Check sheet for the modelled part. Datum: model origin and axes. Units: mm. A direction names the side the tool comes from. Round coordinates to 2 decimals unless told otherwise and drop trailing zeros. Write each loop counter-clockwise with the first axis right and the second up, starting at its lowest first coordinate (ties: lowest second). Pieces come first, ordered by that corner, then holes. Notation, with made-up numbers: (-18.5, -17) -> (30.5, -17) arc R13 ccw to (30.5, 0) -> close; hole circle Ø5 at (88, 31). An arc over 180 degrees is marked (long way). Write item = value, one per line.
from build123d import *

# Parameters (mm, degrees)
F_4_0_4_DURCHMESSER_BOHRUNG1_D     = 4
F_4_0_4_DURCHMESSER_BOHRUNG1_DEPTH = 5.001
KREISMUSTER1_COUNT                 = 4


with BuildPart() as part:
    # Skizze1 → Rotation1 (revolve)
    with BuildSketch(Plane.XY):
        Polygon((0, 12.75), (3, 12.75), (3, 9.75), (23, 7.5), (38, 0), (40, 0), (40, 8), (5, 15.5), (5, 25), (0, 25), align=None)
    revolve(axis=Axis((-34.842488806, 0, 0), (1, 0, 0)))

    # Ø4.0 (4) Durchmesser Bohrung1
    with Locations(Plane.ZY):
        with Locations((-19.44, 0)):
            f_4_0_4_durchmesser_bohrung1 = Hole(F_4_0_4_DURCHMESSER_BOHRUNG1_D / 2, depth=F_4_0_4_DURCHMESSER_BOHRUNG1_DEPTH)

    # Kreismuster1: Ø4.0 (4) Durchmesser Bohrung1 ×4 about axis
    kreismuster1_axis = Axis((0, 0, 0), (1, 0, 0))
    for i in range(1, KREISMUSTER1_COUNT):
        add(f_4_0_4_durchmesser_bohrung1.rotate(kreismuster1_axis, i * 360 / KREISMUSTER1_COUNT), mode=Mode.SUBTRACT)


solid = part.part
(1) Access from +Z, -Z, +X, -X, +Y, -Y to the whole of each face (thin tool, end or side, straight path). Record for faces 1 (the flat face through (40, 0, 0)), 2 (the flat face through (3, 6.6, -7.5)).
Worked answers:
face_1 = +Z, -Z, +X, +Y, -Y
face_2 = -X
(2) Sectioned sample at A-A on y = -19.44. Enter the section's corners in (x, z).
Worked answers:
outline = (0, -15.72) -> (5, -15.72) -> (5, -2) -> (0, -2) -> close; (0, 2) -> (5, 2) -> (5, 15.72) -> (0, 15.72) -> close
(3) Sectioned sample at C-C on x = 18.5. Enter the section's corners in (y, z).
Worked answers:
outline = circle Ø25.21 at (0, 0); hole circle Ø16.01 at (0, 0)
(4) Release check for a two-part mould opening along Y. For faces 3 (the flat face through (5, 11.5, -10.8)), 4 (the conical face through (26.144, 10.463, 3.295)), 5 (the cylindrical face through (2.535, 21.287, -0.766)) record: pulls with the +Y half, pulls with the -Y half, needs draft (parallel to the pull), parting line crosses it, or undercut.
Worked answers:
face_3 = needs draft
face_4 = parting line crosses it
face_5 = undercut
(5) Material ranges on L1, parallel to X at y = -15.5, z = 7; L2, parallel to Z at x = 1.4, y = 19.44, recorded low to high. Write a range as [from, to].
Worked answers:
L1 = [0, 5]
L2 = [-15.72, -2], [2, 15.72]
(6) Go/stop test with flat-tipped pins: P1, Ø2, axis at x = 9, z = -13.5, coming from the +Y side; P2, Ø3, axis at y = -19.44, z = 0, coming from the -X side; P3, Ø12, axis at x = 16, z = 15.5, coming from the -Y side; P4, Ø1, axis at y = 0, z = -16.5, coming from the +X side. Record where each tip stops, or that it passes through.
Worked answers:
P1 = 7.68
P2 = through
P3 = -9.35
P4 = 5
(7) Sectioned sample at D-D on x = 14. Enter the section's corners in (y, z) (1 decimal), then the cut area to 3 significant figures.
Worked answers:
outline = circle Ø27.1 at (0, 0); hole circle Ø17 at (0, 0)
area = 351 mm²
